Design review of the part built by this model. Coordinates are the model's own, in mm. A direction names the side the tool comes from. Coordinates: 2 decimals unless noted, no trailing zeros. Order: outer loops, then holes, each group sorted by start corner. A loop starts at its lowest first (then second) coordinate and runs counter-clockwise, first axis right, second up. Notation, with made-up numbers: (-32, -32) - (-25, -32) arc R37 ccw to (-25, 4) - close; hole circle Ø6 at (4, 19). An arc over 180 degrees is marked (long way). Write each question's results on one line, items separated by ' | '. Start each with the question number.
```python
from build123d import *

# Parameters (mm, degrees)
BOSS_EXTRUDE1_DEPTH = 1.1
BOSS_EXTRUDE2_DEPTH = 3.5


with BuildPart() as part:
    # Sketch1 → Boss-Extrude1 (new body)
    with BuildSketch(Plane(origin=(0, 0, 0), x_dir=(1, 0, 0), z_dir=(0, 1, 0))):
        Polygon((9.705882353, 13.5), (-11.294117647, 13.5), (-11.294117647, -9.5), (-8.294117647, -9.5), (-8.294117647, 10.5), (6.705882353, 10.5), (6.705882353, -9.5), (9.705882353, -9.5), align=None)
    extrude(amount=BOSS_EXTRUDE1_DEPTH)

    # Sketch2 → Boss-Extrude2 (add)
    with BuildSketch(Plane(origin=(0, 1.1, 0), x_dir=(1, 0, 0), z_dir=(0, 1, 0))):
        Polygon((-8.294117647, -9.5), (-5.294117647, -9.5), (-5.294117647, 9.3), (3.705882353, 9.3), (3.705882353, -9.5), (6.705882353, -9.5), (9.705882353, -9.5), (9.705882353, 13.5), (-11.294117647, 13.5), (-11.294117647, -9.5), align=None)
    extrude(amount=BOSS_EXTRUDE2_DEPTH)


solid = part.part
```
(1) Take a section at B-B (y = 2.9). State the section outline as (x, z) points, plus the area to 3 significant figures.
(2) Take a section at A-A (z = 6.25). State the section outline as (x, y) points, plus the area to 3 significant figures.
(3) To check wall thickness, follow line 1 along X through (y, z) = (3.4, -4.25); line 2 along X through (y, z) = (0.85, 6.5); line 3 along Z through (x, y) = (5.5, 0.8). State the ranges of each line that lie inside material, in increasing order. Write a range as [from, to].
(4) Take a section at C-C (x = -3.75). State the section outline as (y, z) points.
(5) Tool access review of faces 4 (the face through (6.706, 0.5, -0.6)), 5 (the face through (-11.294, 2, -2)), 6 (the face through (-5.294, 3, 0)): name each direction out of +Z, -Z, +X, -X, +Y, -Y from which nothing blocks a thin tool from reaching the whole face with its end or side.
(6) Clearance check with flat-ended pins moving along their axes: pin 1 (1 mm diameter, centred on x = -0.5, y = 3, fed in from +Z); pin 2 (3 mm diameter, centred on x = -2.5, z = 6, fed in from +Y). State where each tip first meets the part, or that it passes through.
(7) Take a section at D-D (y = 0.5). State the section outline as (x, z) points.
(8) Mouldability with a two-part tool opening along X and no side actions: class faces 1 (the face through (9.706, 2, -2)), 2 (the face through (4, 1.1, -1)), 3 (the face through (-2, 0, -11)) as +X half, -X half, draft (parallel to the pull), parting line (faces both ways), or undercut.
Worked out:
1) outline: (-11.29, -13.5) - (9.71, -13.5) - (9.71, 9.5) - (3.71, 9.5) - (3.71, -9.3) - (-5.29, -9.3) - (-5.29, 9.5) - (-11.29, 9.5) - close | area: 314 mm^2
2) outline: (-11.29, 0) - (-8.29, 0) - (-8.29, 1.1) - (-5.29, 1.1) - (-5.29, 4.6) - (-11.29, 4.6) - close; (3.71, 1.1) - (6.71, 1.1) - (6.71, 0) - (9.71, 0) - (9.71, 4.6) - (3.71, 4.6) - close | area: 48.6 mm^2
3) line 1: [-11.29, -5.29], [3.71, 9.71] | line 2: [-11.29, -8.29], [6.71, 9.71] | line 3: [-13.5, -10.5]
4) outline: (0, -13.5) - (4.6, -13.5) - (4.6, -9.3) - (1.1, -9.3) - (1.1, -10.5) - (0, -10.5) - close
5) face 4: +Z, -Y | face 5: +Z, -Z, -X, +Y, -Y | face 6: +Z, +Y, -Y
6) pin 1: z = -9.3 | pin 2: through
7) outline: (-11.29, -13.5) - (9.71, -13.5) - (9.71, 9.5) - (6.71, 9.5) - (6.71, -10.5) - (-8.29, -10.5) - (-8.29, 9.5) - (-11.29, 9.5) - close
8) face 1: +X half | face 2: undercut | face 3: draft
